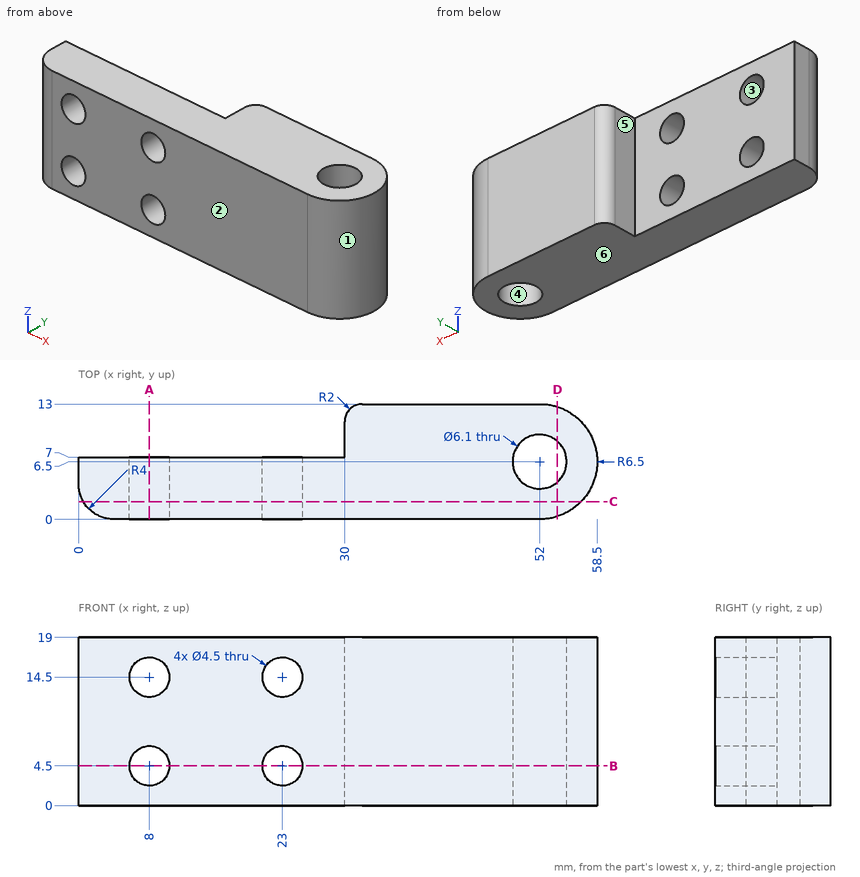
Geometry check sheet. Reference: drawing and pictorial views, mm from the part's lowest x, y, z. A direction names the side the tool comes from. Coordinates: 2 decimals unless noted, no trailing zeros. Order: outer loops, then holes, each group sorted by start corner. A loop starts at its lowest first (then second) coordinate and runs counter-clockwise, first axis right, second up.
Item 1: Section check A-A, the plane x = 8. Enter the section's corners in (y, z).
Filled in:
outline: (0, 0) - (7, 0) - (7, 2.25) - (0, 2.25) - close; (0, 6.75) - (7, 6.75) - (7, 12.25) - (0, 12.25) - close; (0, 16.75) - (7, 16.75) - (7, 19) - (0, 19) - close
Item 2: Depth check by flat-ended pin: pin 1 (2 mm diameter, centred on y = 9, z = 9.5, fed in from +X); pin 2 (1 mm diameter, centred on x = 18, z = 15.5, fed in from +Y). Enter the tip coordinate at first touch or a pass-through.
Filled in:
pin 1: stops at x = 58.32
pin 2: stops at y = 7
Item 3: Access from +Z, -Z, +X, -X, +Y, -Y to the whole of each face (thin tool, end or side, straight path). Record for the marked faces 5 and 6.
Filled in:
face 5: +Z, -Z, -X, +Y
face 6: -Z, +X, -X, +Y, -Y
Item 4: Section check B-B, the plane z = 4.5. Enter the section's corners in (x, y), then the cut area to 3 significant figures.
Filled in:
outline: (0, 4) arc R4 ccw to (4, 0) - (5.75, 0) - (5.75, 7) - (0, 7) - close; (10.25, 0) - (20.75, 0) - (20.75, 7) - (10.25, 7) - close; (25.25, 0) - (52, 0) arc R6.5 ccw to (52, 13) - (32, 13) arc R2 ccw to (30, 11) - (30, 7) - (25.25, 7) - close; hole circle Ø6.1 at (52, 6.5)
area: 466 mm2
Item 5: Material ranges on L1, parallel to Z at x = 8, y = 4.75; L2, parallel to X at y = 2, z = 14.5; L3, parallel to X at y = 1.75, z = 4.75, recorded low to high.
Filled in:
L1: z = 0 to 2.25, 6.75 to 12.25, 16.75 to 19
L2: x = 0.54 to 5.75, 10.25 to 20.75, 25.25 to 56.69
L3: x = 0.69 to 5.76, 10.24 to 20.76, 25.24 to 56.44
Item 6: Section check C-C, the plane y = 2. Enter the section's corners in (x, z).
Filled in:
outline: (0.54, 0) - (56.69, 0) - (56.69, 19) - (0.54, 19) - close; hole circle Ø4.5 at (8, 4.5); hole circle Ø4.5 at (8, 14.5); hole circle Ø4.5 at (23, 4.5); hole circle Ø4.5 at (23, 14.5)
Item 7: Section check D-D, the plane x = 54. Enter the section's corners in (y, z), then the cut area to 3 significant figures.
Filled in:
outline: (0.32, 0) - (4.2, 0) - (4.2, 19) - (0.32, 19) - close; (8.8, 0) - (12.68, 0) - (12.68, 19) - (8.8, 19) - close
area: 148 mm2
Item 8: Release check for a two-part mould opening along Y. For the marked faces 1, 2, 3 and 4 record: +Y half, -Y half, draft (parallel to the pull), parting line (faces both ways), or undercut.
Filled in:
face 1: parting line
face 2: -Y half
face 3: draft
face 4: undercut
